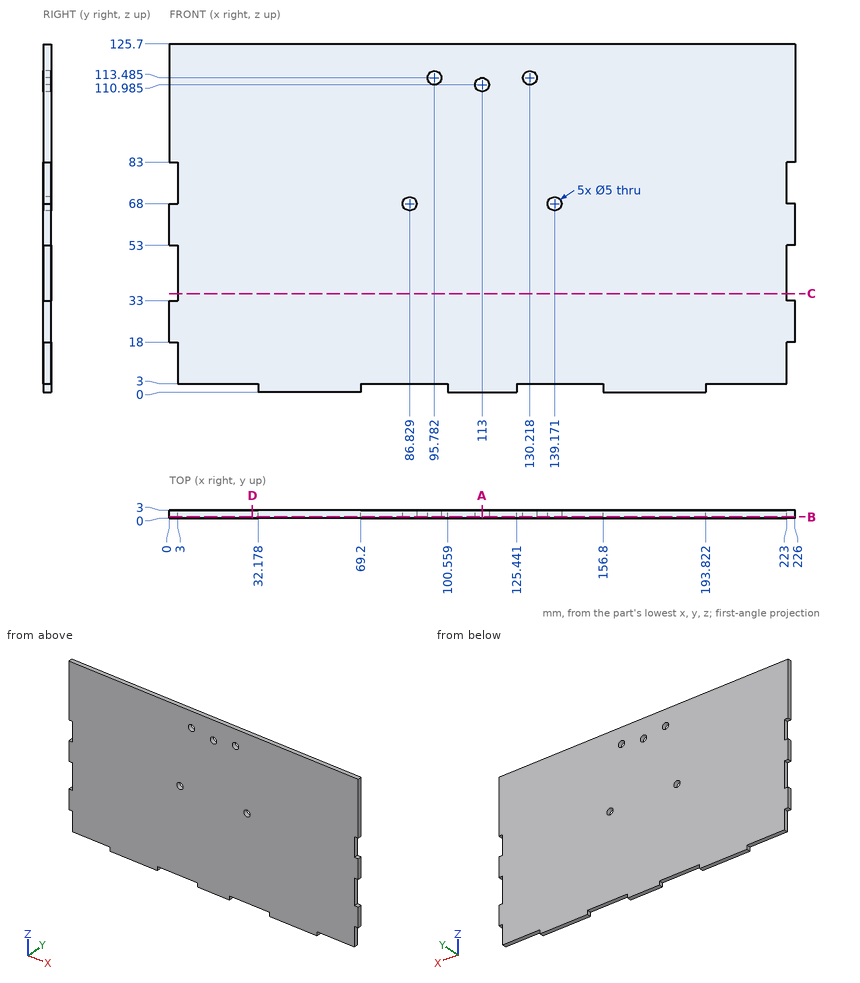
Design review of the part shown in the three views and the two pictorial views. Dimensions are in mm from the part's minimum x, y and z. Give positions to 0.01 mm unless a question says otherwise; leave off trailing zeros. Order: outer loops, then holes, each group sorted by start corner. A loop starts at its lowest first (then second) coordinate and runs counter-clockwise, first axis right, second up. Notation, with made-up numbers: M -25,54 L -18,54 A11 cw -18,64 Z; hole C 20,86 d7. An arc over 180 degrees is marked long. Answer in a Markdown table with one row per item. Add a question column.
(1) For pin 1 (0.9 mm diameter, centred on y = 1.5, z = 12, fed in from +X); pin 2 (0.9 mm diameter, centred on y = 1, z = 1.5, fed in from -X); pin 3 (0.9 mm diameter, centred on x = 1, y = 1.5, fed in from -Z), all flat-tipped, find the tip position at first contact; note any pin that passes through.
(2) Consider section D-D on x = 30. State the section outline as (y, z) points.
(3) Consider section A-A on x = 113. State the section outline as (y, z) points (1 decimal).
(4) Consider section B-B on y = 0.55. Give the number of separate pieces and of enclosed holes in the cut face, and give its area (3 significant figures).
(5) Consider section C-C on z = 35.5. State the section outline as (x, y) points.
(6) Wall thickness on probe 1 along Z at (x, y) = (211, 0.65); probe 2 along X at (y, z) = (0.65, 81.5); probe 3 along Z at (x, y) = (88, 2.55): over which ranges is each line inside the solid? List them lowest first. Write a range as [from, to].
Evaluation:
| question | item | result |
|---|---|---|
| 1 | pin 1 | stops at x = 223 |
| 1 | pin 2 | stops at x = 32.18 |
| 1 | pin 3 | stops at z = 18 |
| 2 | outline | M 0,3 L 3,3 L 3,125.7 L 0,125.7 Z |
| 3 | outline | M 0,0 L 3,0 L 3,108.5 L 0,108.5 Z; M 0,113.5 L 3,113.5 L 3,125.7 L 0,125.7 Z |
| 4 | separate pieces | 1 |
| 4 | enclosed holes | 5 |
| 4 | area | 27,600 mm^2 |
| 5 | outline | M 3,0 L 223,0 L 223,3 L 3,3 Z |
| 6 | probe 1 | z = [3, 125.7] |
| 6 | probe 2 | x = [3, 223] |
| 6 | probe 3 | z = [3, 65.79], [70.21, 125.7] |
